from build123d import *

# Parameters (mm, degrees)
F0_R     = 4
F1_DEPTH = 134.62
F2_R     = 4
F2_R_2   = 2.5
F3_DEPTH = 4
F4_R     = 2.5
F5_DEPTH = 30.48


with BuildPart() as f1:
    # F0 (on Front) → F1 (new body)
    with BuildSketch(Plane.XZ):
        Circle(F0_R)
    extrude(amount=F1_DEPTH)

    # F2 (on face) → F3 (cut)
    with BuildSketch(Plane(origin=(0, 0, 0), x_dir=(-1, 0, 0), z_dir=(0, 1, 0))):
        Circle(F2_R)
        Circle(F2_R_2, mode=Mode.SUBTRACT)
    extrude(amount=-F3_DEPTH, mode=Mode.SUBTRACT)

    # F4 (on face) → F5 (join)
    with BuildSketch(Plane.XZ.offset(134.62)):
        Circle(F4_R)
    extrude(amount=F5_DEPTH)


solid = f1.part
Source: CAD feature listing. Evaluate the final solid. Frame: model axes, mm. A direction names the side the tool comes from. Give positions to 0.01 mm unless a question says otherwise; leave off trailing zeros. Write each loop counter-clockwise with the first axis right and the second up, starting at its lowest first coordinate (ties: lowest second). Pieces come first, ordered by that corner, then holes. Notation, with made-up numbers: (41, -7) - (73, -7) arc R15 cw to (73, 10) - close; hole circle Ø6 at (73, 62.5). An arc over 180 degrees is marked (long way). Write item = value, one per line. Start each with the question number.
Q1. Reachability of faces 1 (the cylindrical face through (-0.54, -149.65, -2.44)), 2 (the flat face through (-2, -4, 2)), 3 (the flat face through (0, -165.1, 0)) from +Z, -Z, +X, -X, +Y, -Y: full face, straight path, thin tool, end or side. Return the list, or none.
Q2. Cut plane C-C, the plane y = -60.5. Return loops of the section in (x, z).
Q3. Pin query (flat end, axial travel): pin 1 Ø1 at (x, y) = (1.5, -40.5) entering from +Z; pin 2 Ø1.5 at (x, y) = (1, -134) entering from +Z; pin 3 Ø1.5 at (y, z) = (-139.5, -1) entering from +X. Return the tip coordinate at first contact, or that it passes through.
Q4. Cut plane D-D, the plane y = -146. Return loops of the section in (x, z).
Q5. Cut plane A-A, the plane x = 0. Return loops of the section in (y, z).
Q6. Material intervals for probe 1 along Y at (x, z) = (2, 3.25); probe 2 along X at (y, z) = (-53.5, -0.5); probe 3 along X at (y, z) = (-123, -3.25), sorted ascending.
Q7. Cut plane B-B, the plane z = 0. Return loops of the section in (x, y).
Computed values:
q1.face_1 = -Y
q1.face_2 = +Y
q1.face_3 = +Z, -Z, +X, -X, -Y
q2.outline = circle Ø8 at (0, 0)
q3.pin_1 = 3.87
q3.pin_2 = 3.99
q3.pin_3 = 2.49
q4.outline = circle Ø5 at (0, 0)
q5.outline = (-165.1, -2.5) - (-134.62, -2.5) - (-134.62, -4) - (-4, -4) - (-4, -2.5) - (0, -2.5) - (0, 2.5) - (-4, 2.5) - (-4, 4) - (-134.62, 4) - (-134.62, 2.5) - (-165.1, 2.5) - close
q6.probe_1 = -134.62 to -4
q6.probe_2 = -3.97 to 3.97
q6.probe_3 = -2.33 to 2.33
q7.outline = (-4, -134.62) - (-2.5, -134.62) - (-2.5, -165.1) - (2.5, -165.1) - (2.5, -134.62) - (4, -134.62) - (4, -4) - (2.5, -4) - (2.5, 0) - (-2.5, 0) - (-2.5, -4) - (-4, -4) - close
